from build123d import *

# Parameters (mm, degrees)
SKETCH1_W               = 5
SKETCH1_H               = 5
SKETCH1_R               = 0.95
CENTER_DEPTH            = 1.3
RIGHTSIDE_START         = 1.3
SKETCH1_2_W             = 5
SKETCH1_2_H             = 5
SKETCH1_2_R             = 0.95
RIGHTSIDE_DEPTH         = 1.2
LEFTSIDE_START          = -1.3
SKETCH1_3_W             = 5
SKETCH1_3_H             = 5
SKETCH1_3_R             = 0.95
LEFTSIDE_DEPTH          = 1.2
SKETCH3_W               = 5
SKETCH3_H               = 5
BOSS_EXTRUDE4_DEPTH     = 47.5
CUT_EXTRUDE1_DEPTH      = 5
CIRPATTERN2_COUNT       = 6
CIRPATTERN3_COUNT       = 3
CIRPATTERN4_START       = -44.601270189
CIRPATTERN4_OUTLINE_W   = 5
CIRPATTERN4_OUTLINE_H   = 5
CIRPATTERN4_OUTLINE_R   = 0.95
CIRPATTERN4_DEPTH       = 2.6
CIRPATTERN4_2_OUTLINE_W = 5
CIRPATTERN4_2_OUTLINE_H = 5
CIRPATTERN4_2_OUTLINE_R = 0.95
CIRPATTERN4_2_DEPTH     = 2.6
CIRPATTERN4_START_2     = -1.3
CIRPATTERN4_3_OUTLINE_W = 5
CIRPATTERN4_3_OUTLINE_H = 5
CIRPATTERN4_3_OUTLINE_R = 0.95
CIRPATTERN4_3_DEPTH     = 2.6
SKETCH5_W               = 5
SKETCH5_H               = 2.6
CUT_EXTRUDE2_DEPTH      = 5


# Read off the part's stored shape, not the designer's step: CirPattern4
with BuildPart() as part:
    # Sketch1 → Center (new, symmetric)
    with BuildSketch(Plane(origin=(0, 0, 0), x_dir=(1, 0, 0), z_dir=(0, 1, 0))):
        Rectangle(SKETCH1_W, SKETCH1_H)
        with Locations(Location((0, 0, 0), (0, 0, 270))):
            Circle(SKETCH1_R, mode=Mode.SUBTRACT)
    extrude(amount=CENTER_DEPTH, both=True)

    # Sketch5 → Cut-Extrude2 (cut)
    with BuildSketch(Plane(origin=(2.5, 0, 0), x_dir=(0, 0, -1), z_dir=(1, 0, 0))):
        Rectangle(SKETCH5_W, SKETCH5_H)
    extrude(amount=-CUT_EXTRUDE2_DEPTH, mode=Mode.SUBTRACT)


with BuildPart() as body_2:
    # Sketch1<2> → RightSide (new body)
    with BuildSketch(Plane(origin=(0, 0, 0), x_dir=(1, 0, 0), z_dir=(0, 1, 0)).offset(RIGHTSIDE_START)):
        Rectangle(SKETCH1_2_W, SKETCH1_2_H)
        with Locations(Location((0, 0, 0), (0, 0, 270))):
            Circle(SKETCH1_2_R, mode=Mode.SUBTRACT)
    extrude(amount=RIGHTSIDE_DEPTH)


with BuildPart() as body_3:
    # Sketch1<3> → LeftSide (new body)
    with BuildSketch(Plane(origin=(0, 0, 0), x_dir=(1, 0, 0), z_dir=(0, 1, 0)).offset(LEFTSIDE_START)):
        Rectangle(SKETCH1_3_W, SKETCH1_3_H)
        with Locations(Location((0, 0, 0), (0, 0, 270))):
            Circle(SKETCH1_3_R, mode=Mode.SUBTRACT)
    extrude(amount=-LEFTSIDE_DEPTH)


with BuildPart() as body_4:
    # Sketch3 → Boss-Extrude4 (new body)
    with BuildSketch(Plane.ZY.offset(2.5)):
        Rectangle(SKETCH3_W, SKETCH3_H)
    extrude(amount=BOSS_EXTRUDE4_DEPTH)

    # Sketch4 → Cut-Extrude1 (cut)
    with BuildSketch(Plane.XY.offset(-2.5)):
        Polygon((-50, 0), (-50, -2.5), (-45.669872981, -2.5), align=None)
        Polygon((-50, 2.5), (-50, 0), (-45.669872981, 2.5), align=None)
    extrude(amount=CUT_EXTRUDE1_DEPTH, mode=Mode.SUBTRACT)


with BuildPart() as cirpattern2_1:
    # CirPattern2: pattern copy
    add(body_4.part.rotate(Axis((-50, 0, 0), (0, 0, 1)), 1 * 360 / CIRPATTERN2_COUNT))


with BuildPart() as cirpattern2_2:
    # CirPattern2: pattern copy
    add(body_4.part.rotate(Axis((-50, 0, 0), (0, 0, 1)), 2 * 360 / CIRPATTERN2_COUNT))


with BuildPart() as cirpattern2_3:
    # CirPattern2: pattern copy
    add(body_4.part.rotate(Axis((-50, 0, 0), (0, 0, 1)), 3 * 360 / CIRPATTERN2_COUNT))


with BuildPart() as cirpattern2_4:
    # CirPattern2: pattern copy
    add(body_4.part.rotate(Axis((-50, 0, 0), (0, 0, 1)), 4 * 360 / CIRPATTERN2_COUNT))


with BuildPart() as cirpattern2_5:
    # CirPattern2: pattern copy
    add(body_4.part.rotate(Axis((-50, 0, 0), (0, 0, 1)), 5 * 360 / CIRPATTERN2_COUNT))


with BuildPart() as cirpattern3_1:
    # CirPattern3: pattern copy
    add(body_3.part.rotate(Axis((-50, 0, 0), (0, 0, 1)), 1 * 360 / CIRPATTERN3_COUNT))


with BuildPart() as cirpattern3_2:
    # CirPattern3: pattern copy
    add(body_3.part.rotate(Axis((-50, 0, 0), (0, 0, 1)), 2 * 360 / CIRPATTERN3_COUNT))


with BuildPart() as cirpattern3_3:
    # CirPattern3: pattern copy
    add(body_2.part.rotate(Axis((-50, 0, 0), (0, 0, 1)), 1 * 360 / CIRPATTERN3_COUNT))


with BuildPart() as cirpattern3_4:
    # CirPattern3: pattern copy
    add(body_2.part.rotate(Axis((-50, 0, 0), (0, 0, 1)), 2 * 360 / CIRPATTERN3_COUNT))


with BuildPart() as body_14:
    # CirPattern4 outline → CirPattern4 (new body)
    with BuildSketch(Plane(origin=(0, 0, 0), x_dir=(0.49999999999999767, 0.86602540378444, 0), z_dir=(0.8660254037844399, -0.49999999999999795, 0)).offset(CIRPATTERN4_START)):
        with Locations((25, 0)):
            Rectangle(CIRPATTERN4_OUTLINE_W, CIRPATTERN4_OUTLINE_H)
        with Locations((25, 0)):
            Circle(CIRPATTERN4_OUTLINE_R, mode=Mode.SUBTRACT)
    extrude(amount=CIRPATTERN4_DEPTH)


with BuildPart() as body_15:
    # CirPattern4 2 outline → CirPattern4 2 (new body)
    with BuildSketch(Plane(origin=(0, 0, 0), x_dir=(0.5000000000000098, -0.8660254037844329, 0), z_dir=(0.8660254037844329, 0.50000000000001, 0)).offset(CIRPATTERN4_START)):
        with Locations((25, 0)):
            Rectangle(CIRPATTERN4_2_OUTLINE_W, CIRPATTERN4_2_OUTLINE_H)
        with Locations((25, 0)):
            Circle(CIRPATTERN4_2_OUTLINE_R, mode=Mode.SUBTRACT)
    extrude(amount=CIRPATTERN4_2_DEPTH)


with BuildPart() as body_16:
    # CirPattern4 3 outline → CirPattern4 3 (new body)
    with BuildSketch(Plane(origin=(0, 0, 0), x_dir=(1, 0, 0), z_dir=(0, 1, 0)).offset(CIRPATTERN4_START_2)):
        with Locations((-100, 0)):
            Rectangle(CIRPATTERN4_3_OUTLINE_W, CIRPATTERN4_3_OUTLINE_H)
        with Locations((-100, 0)):
            Circle(CIRPATTERN4_3_OUTLINE_R, mode=Mode.SUBTRACT)
    extrude(amount=CIRPATTERN4_3_DEPTH)


with BuildPart() as cirpattern2_5_1:
    add(cirpattern2_5.part)

    # Combine1: union CirPattern2_3, CirPattern2_4, body 16, CirPattern3_2, CirPattern3_4, body 15, CirPattern2_1, body 3, body 14, body 4, body 2, CirPattern2_2, CirPattern3_1, CirPattern3_3
    add(cirpattern2_3.part)
    add(cirpattern2_4.part)
    add(body_16.part)
    add(cirpattern3_2.part)
    add(cirpattern3_4.part)
    add(body_15.part)
    add(cirpattern2_1.part)
    add(body_3.part)
    add(body_14.part)
    add(body_4.part)
    add(body_2.part)
    add(cirpattern2_2.part)
    add(cirpattern3_1.part)
    add(cirpattern3_3.part)


solid = cirpattern2_5_1.part
Source: CAD feature listing. Evaluate the final solid. Frame: model axes, mm. A direction names the side the tool comes from. Round coordinates to 2 decimals unless told otherwise and drop trailing zeros. Loops run counter-clockwise (first coordinate to the right, second up) from the corner with the lowest first, then second, coordinate; pieces in that order, holes last.
Q1. Ray query, line 1 (X direction, y = -1.7, z = 0); line 2 (Y direction, x = -55.5, z = -1.7); line 3 (Y direction, x = -32, z = 0.45). Return the intervals inside material, ascending.
Q2. Section A-A, the plane y = 23. Return loops of the section in (x, z), plus the area to 3 significant figures.
Q3. Section B-B, the plane x = -59.5. Return loops of the section in (y, z), plus the area to 3 significant figures.
Q4. Section C-C, the plane x = -80. Return loops of the section in (y, z).
Q5. Access query for faces 1 (the face through (-76.11, 42.62, -1.15)), 2 (the face through (-76, 2.5, 0)), 3 (the face through (-39.06, -23.95, -0.03)). Directions: +Z, -Z, +X, -X, +Y, -Y. A direction counts if a zero-diameter tool reaches every point of the face in a straight line with its end or side. Return the directions, or none.
Q6. Section D-D, the plane z = 0. State how many separate pieces and enclosed holes the cut face has, plus the area to 3 significant figures.
Q7. Mould query, pull axis Y, two halves, no side actions, for faces 4 (the face through (-21, -2.5, 0)), 5 (the face through (-26.7, 42.96, 0.04)), 6 (the face through (-50, 0, -2.5)), 7 (the face through (-23.77, -45.48, 0.03)). Classes: pulls with the +Y half, pulls with the -Y half, needs draft (parallel to the pull), parting line crosses it, or undercut.
Q8. First-contact query: P1, Ø1.5, axis at x = 0, z = 0, coming from the -Y side; P2, Ø2.5, axis at x = -100, z = 0, coming from the +Y side; P3, Ø2.5, axis at x = -0.5, z = -1, coming from the +Y side; P4, Ø2.5, axis at x = -78.5, z = 0.5, coming from the -Y side. Flat tips, straight axial feed; report the tip coordinate or a pass-through.
Solutions:
1. line 1: x = -97.5 to -0.95, 0.95 to 2.5
1. line 2: y = -14.53 to -4.53, -2.5 to 2.5, 4.53 to 14.53
1. line 3: y = -36.18 to -26.18, -2.5 to 2.5, 26.18 to 36.18
2. outline: (-66.17, -2.5) - (-60.39, -2.5) - (-60.39, 2.5) - (-66.17, 2.5) - close; (-39.61, -2.5) - (-33.83, -2.5) - (-33.83, 2.5) - (-39.61, 2.5) - close
2. area: 57.7 mm2
3. outline: (-21.45, -2.5) - (-11.45, -2.5) - (-11.45, 2.5) - (-21.45, 2.5) - close; (-2.5, -2.5) - (2.5, -2.5) - (2.5, 2.5) - (-2.5, 2.5) - close; (11.45, -2.5) - (21.45, -2.5) - (21.45, 2.5) - (11.45, 2.5) - close
3. area: 125 mm2
4. outline: (-2.5, -2.5) - (2.5, -2.5) - (2.5, 2.5) - (-2.5, 2.5) - close
5. face 1: +Z, -Z
5. face 2: +Z, -Z, -X
5. face 3: +Z, -Z, -Y
6. separate pieces: 10
6. enclosed holes: 0
6. area: 1,410 mm2
7. face 4: undercut
7. face 5: pulls with the +Y half
7. face 6: needs draft
7. face 7: pulls with the -Y half
8. P1: passes through
8. P2: stops at y = 1.3
8. P3: stops at y = 2.5
8. P4: stops at y = -44.82
